Verification items for the finished model (mm, model axes). Round coordinates to 2 decimals unless told otherwise and drop trailing zeros. Put each result on its own line as item: value.
from build123d import *

# Parameters (mm, degrees)
SKETCH1_R           = 61.9125
SKETCH1_R_2         = 51.1175
BOSS_EXTRUDE1_DEPTH = 6.35
CHAMFER1_SIZE       = 0.635
CHAMFER2_SIZE       = 0.635
HOLE1_D             = 3.66
HOLE1_DEPTH         = 6.35
CIRPATTERN1_COUNT   = 12
CHAMFER3_SIZE       = 0.635
CHAMFER4_SIZE       = 0.635


with BuildPart() as part:
    # Sketch1 → Boss-Extrude1 (new body)
    with BuildSketch(Plane(origin=(0, 6.35, 0), x_dir=(1, 0, 0), z_dir=(0, 1, 0))):
        Circle(SKETCH1_R)
        Circle(SKETCH1_R_2, mode=Mode.SUBTRACT)
    extrude(amount=-BOSS_EXTRUDE1_DEPTH)

    # Chamfer1
    chamfer1_edges = [part.edges().sort_by_distance(p)[0] for p in [
        (-51.1175, 0, 0),
    ]]
    chamfer(chamfer1_edges, length=CHAMFER1_SIZE)

    # Chamfer2
    chamfer2_edges = [part.edges().sort_by_distance(p)[0] for p in [
        (-51.1175, 6.35, 0),
    ]]
    chamfer(chamfer2_edges, length=CHAMFER2_SIZE)

    # Hole1
    with Locations(Plane(origin=(0, 0, 0), x_dir=(-1, 0, 0), z_dir=(0, -1, 0))):
        with Locations((28.2575, -48.943425695)):
            hole1 = Hole(HOLE1_D / 2, depth=HOLE1_DEPTH)

    # CirPattern1: Hole1 ×12 about axis
    cirpattern1_axis = Axis((0, 0, 0), (0, 1, 0))
    for i in range(1, CIRPATTERN1_COUNT):
        add(hole1.rotate(cirpattern1_axis, i * 360 / CIRPATTERN1_COUNT), mode=Mode.SUBTRACT)

    # Chamfer3
    chamfer3_edges = [part.edges().sort_by_distance(p)[0] for p in [
        (-61.9125, 0, 0),
    ]]
    chamfer(chamfer3_edges, length=CHAMFER3_SIZE)

    # Chamfer4
    chamfer4_edges = [part.edges().sort_by_distance(p)[0] for p in [
        (-61.9125, 6.35, 0),
    ]]
    chamfer(chamfer4_edges, length=CHAMFER4_SIZE)


solid = part.part
Item 1: Release check for a two-part mould opening along X. For faces 1 (the cylindrical face through (-13.42, 3.21, 60.44)), 2 (the flat face through (-37, 6.35, -37)), 3 (the cylindrical face through (27.274, 3.219, -47.4)) record: +X half, -X half, draft (parallel to the pull), parting line (faces both ways), or undercut.
Check sheet entries:
face 1: parting line
face 2: draft
face 3: undercut
Item 2: Section check A-A on z = 0. State how many separate pieces and enclosed holes the cut face has, then the cut area to 3 significant figures.
Check sheet entries:
separate pieces: 4
enclosed holes: 0
area: 89.0 mm^2
Item 3: Gauge pin test, flat ends, axial feed: pin 1 Ø2 at (x, z) = (-28.26, -48.94) entering from +Y; pin 2 Ø4 at (x, z) = (48.94, -28.26) entering from -Y; pin 3 Ø2 at (x, y) = (-11.5, 4) entering from -Z; pin 4 Ø1 at (x, y) = (-0.5, 5) entering from +Z. Record the tip position at first contact, or that the pin passes through.
Check sheet entries:
pin 1: passes through
pin 2: stops at y = 0
pin 3: stops at z = -61.02
pin 4: stops at z = 61.91
Item 4: Material ranges on L1, parallel to Z at x = 1, y = 0.5; L2, parallel to Z at x = 1.5, y = 1; L3, parallel to Z at x = 24, y = 1.5, recorded low to high. Write a range as [from, to].
Check sheet entries:
L1: z = [-61.77, -58.05], [-54.98, -51.24], [51.24, 54.98], [58.05, 61.77]
L2: z = [-61.89, -57.56], [-55.47, -51.1], [51.1, 55.47], [57.56, 61.89]
L3: z = [-57.07, -45.13], [45.13, 57.07]
